from build123d import *

# Parameters (mm, degrees)
SKETCH_1_W          = 300
SKETCH_1_H          = 12
EXTRUDE_320_DEPTH   = 17.35
SKETCH_2_W          = 300
SKETCH_2_H          = 1
CUT_EXTRUDE_1_DEPTH = 1
SKETCH_5_R          = 3
CUT_EXTRUDE_6_DEPTH = 152.476144987


with BuildPart() as part:
    # Эскиз1 → Extrude 320 (new body)
    with BuildSketch(Plane(origin=(0, 0, 0), x_dir=(1, 0, 0), z_dir=(0, 1, 0))):
        with Locations((0, 6)):
            Rectangle(SKETCH_1_W, SKETCH_1_H)
    extrude(amount=EXTRUDE_320_DEPTH)

    # Эскиз2 → Вырез-Вытянуть1 (cut)
    with BuildSketch(Plane(origin=(0, 17.35, 0), x_dir=(1, 0, 0), z_dir=(0, 1, 0))):
        with Locations((0, 0.5)):
            Rectangle(SKETCH_2_W, SKETCH_2_H)
    extrude(amount=-CUT_EXTRUDE_1_DEPTH, mode=Mode.SUBTRACT)

    # Эскиз5 → Валы-6мм (cut, through all)
    with BuildSketch(Plane.XY):
        with Locations((-144, 8.175)):
            Circle(SKETCH_5_R)
        with Locations((144, 8.175)):
            Circle(SKETCH_5_R)
    extrude(amount=-CUT_EXTRUDE_6_DEPTH, mode=Mode.SUBTRACT)

    # Эскиз10 → Фиксация-M4 (revolve, cut)
    with BuildSketch(Plane(origin=(150, 8.175, -6), x_dir=(0, 0, -1), z_dir=(0, 1, 0))):
        Polygon((0, 0), (0, 10.991420021), (1.65, 10), (1.65, 0), align=None)
    hole_wizard_m4 = revolve(axis=Axis((156.35, 8.175, -6), (-1, 0, 0)), mode=Mode.SUBTRACT)

    # Зеркальное отражение1: Фиксация-M4 across plane
    add(hole_wizard_m4.mirror(Plane(origin=(0, 0, 0), x_dir=(0, 0, 1), z_dir=(1, 0, 0))), mode=Mode.SUBTRACT)


solid = part.part
Design review of the part built by this model. Coordinates are the model's own, in mm. Give positions to 0.01 mm unless a question says otherwise; leave off trailing zeros. Write each loop counter-clockwise with the first axis right and the second up, starting at its lowest first coordinate (ties: lowest second). Pieces come first, ordered by that corner, then holes. Notation, with made-up numbers: M 56.25,-0.75 L 73.25,-0.75 A23 cw 73.25,11.25 Z; hole C 66.25,32 d4. An arc over 180 degrees is marked long. Return JSON: item names as keys, results as strings. Group by question number.
Item 1: Clearance check with flat-ended pins moving along their axes: pin 1 Ø0.8 at (x, z) = (24.5, -0.5) entering from +Y; pin 2 Ø3 at (y, z) = (8.175, -6) entering from -X. State where each tip first meets the part, or that it passes through.
Item 2: The part is to be moulded in two halves that separate along X. For faces 1 (the flat face through (-2, 8, 0)), 2 (the cylindrical face through (145.38, 5.51, -5.92)), 3 (the flat face through (-150, 10, -6)), 4 (the cylindrical face through (-142.62, 5.51, -5.92)), say which applies: pulls with the +X half, pulls with the -X half, needs draft (parallel to the pull), parting line crosses it, or undercut.
Item 3: Wall thickness on line 1 along Y through (x, z) = (149.3, -6) (3 decimals); line 2 along X through (y, z) = (5.75, -7.5); line 3 along X through (y, z) = (9.75, -5.75): over which ranges is each line inside the solid? List them lowest first.
Item 4: Take a section at A-A (x = 144). Give the boundary of the cut face in (y, z) (3 decimals).
Return value:
{
 "1": {"pin 1": "stops at y = 16.35", "pin 2": "stops at x = -139.91"},
 "2": {"face 1": "needs draft", "face 2": "undercut", "face 3": "pulls with the -X half", "face 4": "undercut"},
 "3": {"line 1": "y = 0 to 6.525, 9.825 to 17.35", "line 2": "x = -150 to -145.77, -142.23 to 142.23, 145.77 to 150", "line 3": "x = -139.97 to 139.97"},
 "4": {"outline": "M 0,-12 L 5.175,-12 L 5.175,0 L 0,0 Z; M 11.175,-12 L 17.35,-12 L 17.35,-1 L 16.35,-1 L 16.35,0 L 11.175,0 Z"}
}
